Source: CAD feature listing. Evaluate the final solid. Frame: model axes, mm. Face numbers are marked on the shaded views. A direction names the side the tool comes from. Coordinates: 2 decimals unless noted, no trailing zeros. Order: outer loops, then holes, each group sorted by start corner. A loop starts at its lowest first (then second) coordinate and runs counter-clockwise, first axis right, second up. Notation, with made-up numbers: (83, -32) -> (120, -32) arc R30 ccw to (120, 0) -> close; hole circle Ø11 at (13.25, 4). An arc over 180 degrees is marked (long way). Put each result on its own line as item: value.
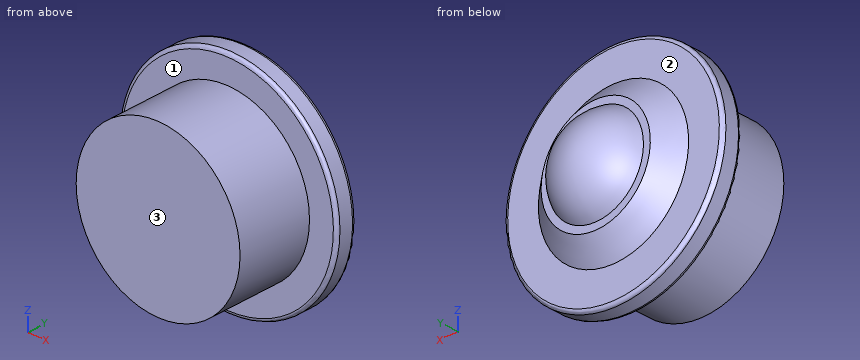
from build123d import *

# Parameters (mm, degrees)
CONG_1_R = 0.5


with BuildPart() as part:
    # Esquisse1 → Révolution1 (revolve)
    with BuildSketch(Plane.XY, mode=Mode.PRIVATE) as r_volution1_sk:
        with BuildLine():
            Line((0, 0), (-12, 0))
            Line((-12, 0), (-12, 11))
            Line((-12, 11), (-16, 11))
            Line((-16, 11), (-16, 14))
            Line((-16, 14), (-11, 14))
            Line((-11, 14), (-8, 16.821458712))
            Line((-8, 16.821458712), (-6.992498005, 16.821458712))
            ThreePointArc((-6.992498005, 16.821458712), (-4.072936154, 19.875775164), (0, 21))
            Line((0, 21), (0, 0))
        make_face()
    revolve(r_volution1_sk.sketch.rotate(Axis((0, 0, 0), (0, 1, 0)), 270), axis=Axis((0, 0, 0), (0, 1, 0)))

    # Congé1
    cong_1_edges = [part.edges().sort_by_distance(p)[0] for p in [
        (0, 11, 16),
        (0, 14, 16),
    ]]
    fillet(cong_1_edges, radius=CONG_1_R)


solid = part.part
1. Cut plane C-C on y = 9.25. Output: boundary loops of the cut face in (x, z), plus the area to 3 significant figures.
Numbers:
outline: circle Ø24 at (0, 0)
area: 452 mm2
2. Cut plane A-A on z = 0. Output: boundary loops of the cut face in (x, y).
Numbers:
outline: (-16, 11.5) arc R0.5 ccw to (-15.5, 11) -> (-12, 11) -> (-12, 0) -> (12, 0) -> (12, 11) -> (15.5, 11) arc R0.5 ccw to (16, 11.5) -> (16, 13.5) arc R0.5 ccw to (15.5, 14) -> (11, 14) -> (8, 16.82) -> (6.99, 16.82) arc R7.94 ccw to (-6.99, 16.82) -> (-8, 16.82) -> (-11, 14) -> (-15.5, 14) arc R0.5 ccw to (-16, 13.5) -> close
3. Ray query, line 1 along Y through (x, z) = (2, 14); line 2 along Z through (x, y) = (3.5, 6); line 3 along Y through (x, z) = (-4, -1.5). Return the intervals inside material, ascending.
Numbers:
line 1: y = 11 to 14
line 2: z = -11.48 to 11.48
line 3: y = 0 to 19.75
4. Cut plane D-D on y = 16. Output: boundary loops of the cut face in (x, z), plus the area to 3 significant figures.
Numbers:
outline: circle Ø17.75 at (0, 0)
area: 247 mm2
5. Set-up query: the marked faces 1, 2 and 3. Return all of +Z, -Z, +X, -X, +Y, -Y with unobstructed straight access to the full face (end or side cutting, diameter ignored); none if empty.
Numbers:
face 1: -Y
face 2: +Y
face 3: +Z, -Z, +X, -X, -Y
6. Cut plane B-B on x = 0. Output: boundary loops of the cut face in (y, z), plus the area to 3 significant figures.
Numbers:
outline: (0, -12) -> (11, -12) -> (11, -15.5) arc R0.5 ccw to (11.5, -16) -> (13.5, -16) arc R0.5 ccw to (14, -15.5) -> (14, -11) -> (16.82, -8) -> (16.82, -6.99) arc R7.94 ccw to (16.82, 6.99) -> (16.82, 8) -> (14, 11) -> (14, 15.5) arc R0.5 ccw to (13.5, 16) -> (11.5, 16) arc R0.5 ccw to (11, 15.5) -> (11, 12) -> (0, 12) -> close
area: 455 mm2
7. First-contact query: pin 1 (6 mm diameter, centred on x = 9.5, y = 7.5, fed in from -Z); pin 2 (12 mm diameter, centred on x = 8.5, y = 8.5, fed in from -Z); pin 3 (6 mm diameter, centred on x = 9.5, z = -2.5, fed in from +Y); pin 4 (1 mm diameter, centred on x = 6, z = 1, fed in from -Y). Flat tips, straight axial feed; report the tip coordinate or a pass-through.
Numbers:
pin 1: stops at z = -10.09
pin 2: stops at z = -15.66
pin 3: stops at y = 17.12
pin 4: stops at y = 0
